Job drawing, mm, ordinate dimensions from the low corner. One solid piece. Give positions to 0.01 mm unless a question says otherwise; leave off trailing zeros. Order: outer loops, then holes, each group sorted by start corner. A loop starts at its lowest first (then second) coordinate and runs counter-clockwise, first axis right, second up. Notation, with made-up numbers: (63.25, 29.25) -> (118.25, 29.25) arc R16 cw to (118.25, 57.25) -> close; hole circle Ø10 at (36, 36). An arc over 180 degrees is marked (long way). Use CSV: the item, a comma, the result in double quotes. Start each with the question number.
1. Cut at B-B on y = 15. List the corners of the cut face in (x, z).
2. Wall check: line 1 (Y direction, x = 18, z = 21); line 2 (Z direction, x = 15, y = 12.25); line 3 (Y direction, x = 37.75, z = 16.5). Give the ranges that are in metal, low to high. Write a range as from..to.
3. Cut at C-C on x = 9.5. List the corners of the cut face in (y, z), then the cut area to 3 significant figures.
4. Cut at D-D on z = 16.5. List the corners of the cut face in (x, y), then the cut area to 3 significant figures.
5. Pull direction Z, two halves, no side cores. Call the marked faces 1, 2, 3 and 4: released by +Z, released by -Z, zero draft, split by the parting line, or undercut.
6. Cut at A-A on z = 12. List the corners of the cut face in (x, y), then the cut area to 3 significant figures.
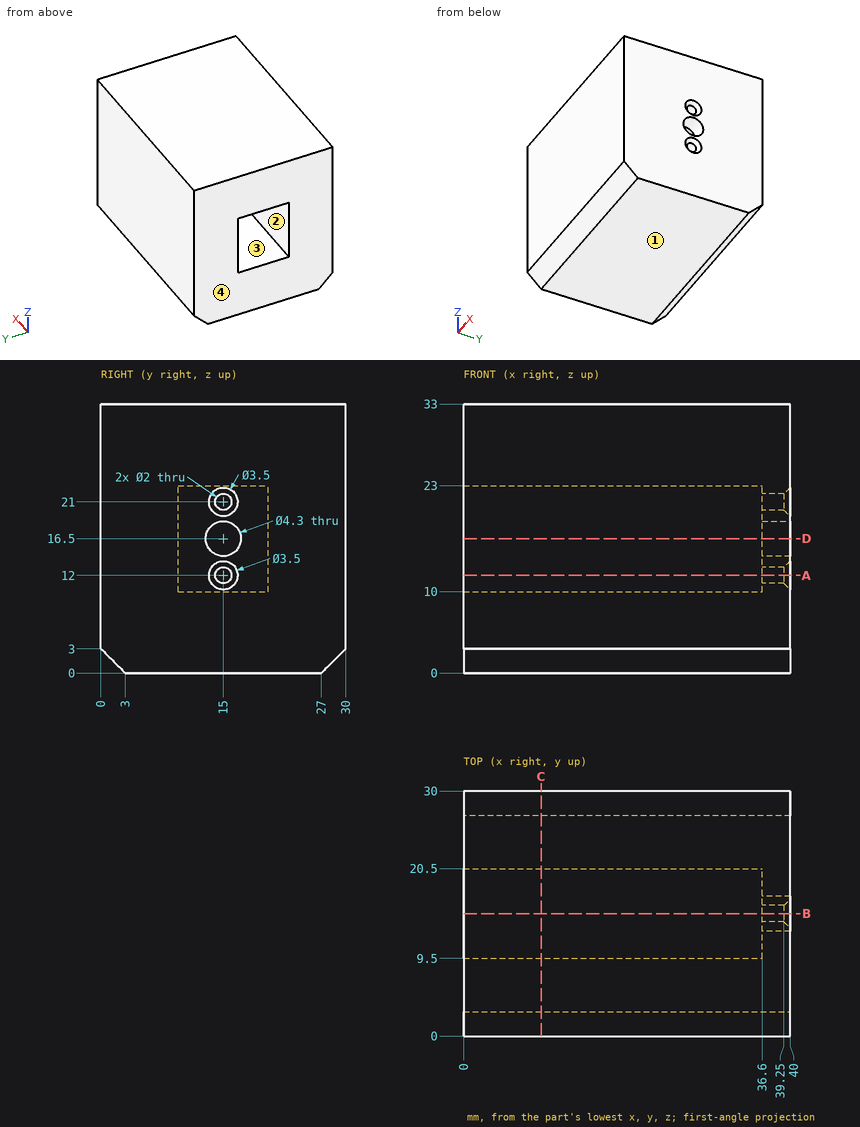
Verdict:
1,outline,"(0, 0) -> (40, 0) -> (40, 10.25) -> (39.25, 11) -> (36.6, 11) -> (36.6, 10) -> (0, 10) -> close; (0, 23) -> (36.6, 23) -> (36.6, 22) -> (39.25, 22) -> (40, 22.75) -> (40, 33) -> (0, 33) -> close; (36.6, 13) -> (39.25, 13) -> (40, 13.75) -> (40, 14.35) -> (36.6, 14.35) -> close; (36.6, 18.65) -> (40, 18.65) -> (40, 19.25) -> (39.25, 20) -> (36.6, 20) -> close"
2,line 1,"0..9.5, 20.5..30"
2,line 2,"0..10, 23..33"
2,line 3,"0..12.85, 17.15..30"
3,outline,"(0, 3) -> (3, 0) -> (27, 0) -> (30, 3) -> (30, 33) -> (0, 33) -> close; hole (9.5, 10) -> (20.5, 10) -> (20.5, 23) -> (9.5, 23) -> close"
3,area,"838 mm^2"
4,outline,"(0, 0) -> (40, 0) -> (40, 12.85) -> (36.6, 12.85) -> (36.6, 9.5) -> (0, 9.5) -> close; (0, 20.5) -> (36.6, 20.5) -> (36.6, 17.15) -> (40, 17.15) -> (40, 30) -> (0, 30) -> close"
4,area,"783 mm^2"
5,face 1,"released by -Z"
5,face 2,"undercut"
5,face 3,"undercut"
5,face 4,"zero draft"
6,outline,"(0, 0) -> (40, 0) -> (40, 13.25) -> (39.25, 14) -> (36.6, 14) -> (36.6, 9.5) -> (0, 9.5) -> close; (0, 20.5) -> (36.6, 20.5) -> (36.6, 16) -> (39.25, 16) -> (40, 16.75) -> (40, 30) -> (0, 30) -> close"
6,area,"790 mm^2"
